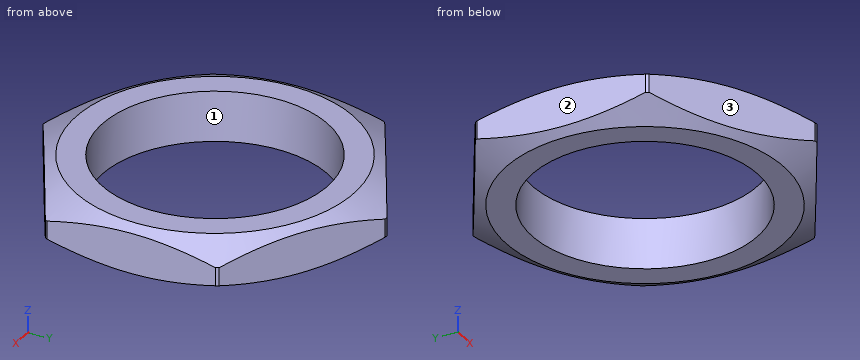
```python
from build123d import *

# Parameters (mm, degrees)
SKETCH_3_R          = 8.5
SKETCH_3_R_2        = 5.6
EXTRUDE_2_DEPTH     = 2.5
CHAMFER_1_SIZE      = 0.8
CHAMFER_1_SIZE2     = 1.6
CHAMFER_2_SIZE      = 1.6
CHAMFER_2_SIZE2     = 0.8
SKETCH_4_OUTSIDE_W  = 23.834
SKETCH_4_OUTSIDE_H  = 23.834
CUT_EXTRUDE_3_DEPTH = 13.278029158


with BuildPart() as part:
    # Эскиз3 → Вытянуть2 (new body)
    with BuildSketch(Plane.XY):
        Circle(SKETCH_3_R)
        Circle(SKETCH_3_R_2, mode=Mode.SUBTRACT)
    extrude(amount=EXTRUDE_2_DEPTH)

    # Фаска1
    chamfer_1_edges = [part.edges().sort_by_distance(p)[0] for p in [
        (-8.5, 0, 2.5),
    ]]
    chamfer_1_side = [part.faces().sort_by_distance(p)[0] for p in [
        (-8.5, 0, 1.25),
    ]]
    chamfer(chamfer_1_edges, length=CHAMFER_1_SIZE, length2=CHAMFER_1_SIZE2, reference=chamfer_1_side[0])

    # Фаска2
    chamfer_2_edges = [part.edges().sort_by_distance(p)[0] for p in [
        (-8.5, 0, 0),
    ]]
    chamfer_2_side = [part.faces().sort_by_distance(p)[0] for p in [
        (-8.259583694, 0, 0),
    ]]
    chamfer(chamfer_2_edges, length=CHAMFER_2_SIZE, length2=CHAMFER_2_SIZE2, reference=chamfer_2_side[0])

    # Эскиз4 outside → Вытянуть3 (cut, through all)
    with BuildSketch(Plane.XY.offset(2.5)):
        Rectangle(SKETCH_4_OUTSIDE_W, SKETCH_4_OUTSIDE_H)
        Polygon((0, 8.544783984), (-7.4, 4.272391992), (-7.4, -4.272391992), (0, -8.544783984), (7.4, -4.272391992), (7.4, 4.272391992), align=None, mode=Mode.SUBTRACT)
    extrude(amount=-CUT_EXTRUDE_3_DEPTH, mode=Mode.SUBTRACT)


solid = part.part
```
Part model, mm, in its own coordinate system. Face numbers are marked on the shaded views. Coordinates: 2 decimals unless noted, no trailing zeros. Write each loop counter-clockwise with the first axis right and the second up, starting at its lowest first coordinate (ties: lowest second). Pieces come first, ordered by that corner, then holes.
Item 1: Slice it at B-B (z = 2.05). Write the cut outline in (x, y).
Item 2: Probe line 1 (Y direction, x = 0, z = 1); line 2 (Y direction, x = 3, z = 1.3); line 3 (X direction, y = -4, z = 1.65). List the from-to ranges inside material, lowest first.
Item 3: Pin check, flat tips, straight feed: pin 1 (5 mm diameter, centred on x = -1.5, y = -4.5, fed in from -Z); pin 2 (1 mm diameter, centred on x = -3.5, z = 1, fed in from -Y). Stop position of each tip, or through.
Item 4: Mould opens along Y. For the marked faces 1, 2 and 3 say: released by +Y, released by -Y, zero draft, split by the parting line, or undercut.
Item 5: Slice it at A-A (y = 0). Write the cut outline in (x, z).
Results found:
1. outline: (-7.4, -2.47) arc R7.8 ccw to (-5.84, -5.18) - (-1.56, -7.64) arc R7.8 ccw to (1.56, -7.64) - (5.84, -5.18) arc R7.8 ccw to (7.4, -2.47) - (7.4, 2.47) arc R7.8 ccw to (5.84, 5.18) - (1.56, 7.64) arc R7.8 ccw to (-1.56, 7.64) - (-5.84, 5.18) arc R7.8 ccw to (-7.4, 2.47) - close; hole circle Ø11.2 at (0, 0)
2. line 1: y = -8.5 to -5.6, 5.6 to 8.5
2. line 2: y = -6.81 to -4.73, 4.73 to 6.81
2. line 3: x = -7.4 to -3.92, 3.92 to 7.4
3. pin 1: stops at z = 0
3. pin 2: stops at y = -6.81
4. face 1: undercut
4. face 2: zero draft
4. face 3: released by -Y
5. outline: (-7.4, 0.25) - (-6.9, 0) - (-5.6, 0) - (-5.6, 2.5) - (-6.9, 2.5) - (-7.4, 2.25) - close; (5.6, 0) - (6.9, 0) - (7.4, 0.25) - (7.4, 2.25) - (6.9, 2.5) - (5.6, 2.5) - close
